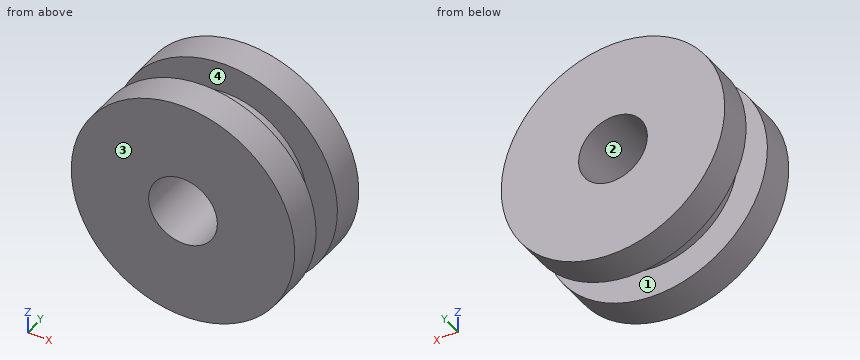
from build123d import *

# Parameters (mm, degrees)
SKETCH_1_R               = 6.5
SKETCH_1_R_2             = 2
EXTRUDE_1_DEPTH          = 6
CUT_EXTRUDE_1_DEPTH      = 1
CUT_EXTRUDE_1_DEPTH_BACK = 1
SKETCH_4_R               = 7
SKETCH_4_R_2             = 4.75


with BuildPart() as part:
    # 草图1 → 凸台-拉伸1 (new body)
    with BuildSketch(Plane(origin=(0, 0, 0), x_dir=(1, 0, 0), z_dir=(0, 1, 0))):
        with Locations(Location((0, 0, 0), (0, 0, 270))):
            Circle(SKETCH_1_R)
        with Locations(Location((0, 0, 0), (0, 0, 270))):
            Circle(SKETCH_1_R_2, mode=Mode.SUBTRACT)
    extrude(amount=EXTRUDE_1_DEPTH)

    # 草图4 → 切除-拉伸1 (cut, two sides: drawn at the far end of the back side and taken through both)
    with BuildSketch(Plane(origin=(0, 3, 0), x_dir=(1, 0, 0), z_dir=(0, 1, 0)).offset(-CUT_EXTRUDE_1_DEPTH_BACK)):
        Circle(SKETCH_4_R)
        with Locations(Location((0, 0, 0), (0, 0, 270))):
            Circle(SKETCH_4_R_2, mode=Mode.SUBTRACT)
    extrude(amount=CUT_EXTRUDE_1_DEPTH + CUT_EXTRUDE_1_DEPTH_BACK, mode=Mode.SUBTRACT)


solid = part.part
The model under review builds one solid part; all positions refer to its coordinate system, in mm. Face numbers are marked on the shaded views. Coordinates: 2 decimals unless noted, no trailing zeros. Write each loop counter-clockwise with the first axis right and the second up, starting at its lowest first coordinate (ties: lowest second). Pieces come first, ordered by that corner, then holes. Notation, with made-up numbers: (-20, 55.5) - (39, 55.5) arc R28 cw to (39, 87.5) - close; hole circle Ø8 at (-12.5, 16.5). An arc over 180 degrees is marked (long way). Answer as a JSON object with one key per item and string values. Group by question number.
1. To check wall thickness, follow probe 1 along X at (y, z) = (4.4, 0); probe 2 along Y at (x, z) = (-3.25, 5); probe 3 along X at (y, z) = (2.2, 0). State the ranges of each line that lie inside material, in increasing order.
2. Add section D-D (z = -2.75). Give the boundary of the cut face in (x, y).
3. Add section B-B (z = 0). Give the boundary of the cut face in (x, y).
4. Add section C-C (y = 4.2). Give the boundary of the cut face in (x, z).
5. Clearance check with a flat-ended pin moving along its axis: pin 1 Ø3 at (x, y) = (-3.5, 1) entering from +Z. State where the tip first meets the part, or that it passes through.
6. Add section A-A (x = 0). Give the boundary of the cut face in (y, z), plus the area to 3 significant figures.
7. Mouldability with a two-part tool opening along Y and no side actions: class the marked faces 1, 2, 3 and 4 as pulls with the +Y half, pulls with the -Y half, needs draft (parallel to the pull), parting line crosses it, or undercut.
Findings:
{
 "1": {"probe 1": "-6.5 to -2, 2 to 6.5", "probe 2": "0 to 2, 4 to 6", "probe 3": "-4.75 to -2, 2 to 4.75"},
 "2": {"outline": "(-5.89, 0) - (5.89, 0) - (5.89, 2) - (3.87, 2) - (3.87, 4) - (5.89, 4) - (5.89, 6) - (-5.89, 6) - (-5.89, 4) - (-3.87, 4) - (-3.87, 2) - (-5.89, 2) - close"},
 "3": {"outline": "(-6.5, 0) - (-2, 0) - (-2, 6) - (-6.5, 6) - (-6.5, 4) - (-4.75, 4) - (-4.75, 2) - (-6.5, 2) - close; (2, 0) - (6.5, 0) - (6.5, 2) - (4.75, 2) - (4.75, 4) - (6.5, 4) - (6.5, 6) - (2, 6) - close"},
 "4": {"outline": "circle Ø13 at (0, 0); hole circle Ø4 at (0, 0)"},
 "5": {"pin 1": "z = 6.18"},
 "6": {"outline": "(0, -6.5) - (2, -6.5) - (2, -4.75) - (4, -4.75) - (4, -6.5) - (6, -6.5) - (6, -2) - (0, -2) - close; (0, 2) - (6, 2) - (6, 6.5) - (4, 6.5) - (4, 4.75) - (2, 4.75) - (2, 6.5) - (0, 6.5) - close", "area": "47.0 mm²"},
 "7": {"face 1": "undercut", "face 2": "needs draft", "face 3": "pulls with the -Y half", "face 4": "undercut"}
}
